Geometry check sheet. Reference: the model listing, model coordinates, mm. A direction names the side the tool comes from. Round coordinates to 2 decimals unless told otherwise and drop trailing zeros. Write each loop counter-clockwise with the first axis right and the second up, starting at its lowest first coordinate (ties: lowest second). Pieces come first, ordered by that corner, then holes. Notation, with made-up numbers: M 8.25,10.25 L 66.25,10.25 A25 ccw 66.25,29.25 Z; hole C 61.5,10 d11. An arc over 180 degrees is marked long. Use a Markdown table: item, result.
```python
from build123d import *

# Parameters (mm, degrees)
BOSS_EXTRUDE1_DEPTH  = 1.5875
M4_CLEARANCE_HOLE1_D = 4.5
BOSS_EXTRUDE2_DEPTH  = 3.175
M3_CLEARANCE_HOLE1_D = 3.4
FILLET1_R            = 3.5
SKETCH8_R            = 2.15
CUT_EXTRUDE1_DEPTH   = 4.1750001
SKETCH9_R            = 2.75
SKETCH9_R_2          = 2.15
BOSS_EXTRUDE3_DEPTH  = 0.75
SKETCH11_R           = 3.5
CUT_EXTRUDE2_DEPTH   = 2.5
SKETCH12_R           = 2.75
CUT_EXTRUDE3_DEPTH   = 0.2
SKETCH13_R           = 3
SKETCH13_R_2         = 2.25
BOSS_EXTRUDE5_DEPTH  = 1.5


with BuildPart() as part:
    # Sketch2 → Boss-Extrude1 (new body, symmetric)
    with BuildSketch(Plane.XY):
        with BuildLine():
            add(Edge.make_bspline(
                [(-24.777431429, -6.350183234), (-24.299810251, -5.902972393), (-23.32289496, -5.01651393), (-22.058866471, -3.944003435), (-21.276036232, -3.316259916), (-20.98344634, -3.086723573)],
                knots=[0, 0, 0, 0, 0.03125, 0.0625, 0.081068463, 0.081068463, 0.081068463, 0.081068463], degree=3))
            Line((-24.777431429, -6.350183234), (-21.36, -10))
            add(Edge.make_bspline(
                [(-21.36, -10), (-20.09052587, -8.81135381), (-18.821051739, -7.728673603), (-17.551577609, -6.751959378)],
                knots=[0, 0, 0, 0, 0.089148464, 0.089148464, 0.089148464, 0.089148464], degree=3))
            Line((-17.551577609, -6.751959378), (-20.98344634, -3.086723573))
        make_face()
        with BuildLine():
            Line((-21.36, -10), (-24.777431429, -6.350183234))
            ThreePointArc((-24.777431429, -6.350183234), (-26.357299125, -9.8356788), (-25.009816701, -13.417431499))
            ThreePointArc((-25.009816701, -13.417431499), (-21.5243212, -14.997299125), (-17.942568571, -13.649816766))
            Line((-17.942568571, -13.649816766), (-21.36, -10))
        make_face()
        with BuildLine():
            ThreePointArc((-25.009816701, -13.417431499), (-26.357299125, -9.8356788), (-24.777431429, -6.350183234))
            add(Edge.make_bspline(
                [(-24.777431429, -6.350183234), (-24.299810251, -5.902972393), (-23.32289496, -5.01651393), (-22.058866471, -3.944003435), (-21.276036232, -3.316259916), (-20.98344634, -3.086723573)],
                knots=[0, 0, 0, 0, 0.03125, 0.0625, 0.081068463, 0.081068463, 0.081068463, 0.081068463], degree=3))
            Line((-20.98344634, -3.086723573), (-21.127614663, -2.932751805))
            Line((-21.127614663, -2.932751805), (-23.519816663, -0.377880068))
            ThreePointArc((-23.519816663, -0.377880068), (-30.587064859, -0.145494731), (-30.819450196, -7.212742926))
            Line((-30.819450196, -7.212742926), (-28.427248195, -9.767614663))
            Line((-28.427248195, -9.767614663), (-25.009816701, -13.417431499))
        make_face()
        with BuildLine():
            add(Edge.make_bspline(
                [(-21.36, -10), (-20.09052587, -8.81135381), (-18.821051739, -7.728673603), (-17.551577609, -6.751959378)],
                knots=[0, 0, 0, 0, 0.089148464, 0.089148464, 0.089148464, 0.089148464], degree=3))
            Line((-21.36, -10), (-17.942568571, -13.649816766))
            add(Edge.make_bspline(
                [(-17.942568571, -13.649816766), (-17.543072686, -13.275756949), (-16.7212792, -12.530114496), (-15.44829951, -11.450473224), (-14.582019434, -10.770813046), (-14.116024052, -10.421130577)],
                knots=[0, 0, 0, 0, 0.03125, 0.0625, 0.099339971, 0.099339971, 0.099339971, 0.099339971], degree=3))
            Line((-14.116024052, -10.421130577), (-14.292751805, -10.232385337))
            Line((-14.292751805, -10.232385337), (-17.551577609, -6.751959378))
        make_face()
        with BuildLine():
            ThreePointArc((-17.942568571, -13.649816766), (-21.5243212, -14.997299125), (-25.009816701, -13.417431499))
            Line((-25.009816701, -13.417431499), (-21.592385337, -17.067248195))
            Line((-21.592385337, -17.067248195), (-19.200183337, -19.622119932))
            ThreePointArc((-19.200183337, -19.622119932), (-12.132935141, -19.854505269), (-11.900549804, -12.787257074))
            Line((-11.900549804, -12.787257074), (-14.116024052, -10.421130577))
            add(Edge.make_bspline(
                [(-17.942568571, -13.649816766), (-17.543072686, -13.275756949), (-16.7212792, -12.530114496), (-15.44829951, -11.450473224), (-14.582019434, -10.770813046), (-14.116024052, -10.421130577)],
                knots=[0, 0, 0, 0, 0.03125, 0.0625, 0.099339971, 0.099339971, 0.099339971, 0.099339971], degree=3))
        make_face()
        with BuildLine():
            add(Edge.make_bspline(
                [(-20.98344634, -3.086723573), (-20.291201445, -2.543658465), (-18.603117827, -1.28817338), (-15.885096675, 0.462779531), (-11.785009924, 2.624744664), (-6.509375137, 4.48808894), (0, 5.25595553), (6.509375137, 4.48808894), (11.785009924, 2.624744664), (15.885096675, 0.462779531), (18.901874802, -1.480633029), (21.37388106, -3.362802893), (23.32289496, -5.01651393), (24.299810251, -5.902972393), (24.777431429, -6.350183234)],
                knots=[0.081068463, 0.081068463, 0.081068463, 0.081068463, 0.125, 0.1875, 0.25, 0.375, 0.5, 0.625, 0.75, 0.8125, 0.875, 0.9375, 0.96875, 1, 1, 1, 1], degree=3))
            Line((-20.98344634, -3.086723573), (-17.551577609, -6.751959378))
            Line((-17.551577609, -6.751959378), (-14.292751805, -10.232385337))
            Line((-14.292751805, -10.232385337), (-14.116024052, -10.421130577))
            add(Edge.make_bspline(
                [(-14.116024052, -10.421130577), (-13.791445759, -10.177567349), (-12.680801028, -9.370838959), (-10.815202086, -8.171392792), (-7.794818062, -6.582915934), (-4.170679183, -5.321481205), (0, -4.839259398), (4.170679183, -5.321481205), (7.794818062, -6.582915934), (10.815202086, -8.171392792), (13.136984474, -9.664132159), (15.119482265, -11.171596294), (16.7212792, -12.530114496), (17.543072686, -13.275756949), (17.942568571, -13.649816766)],
                knots=[0.099339971, 0.099339971, 0.099339971, 0.099339971, 0.125, 0.1875, 0.25, 0.375, 0.5, 0.625, 0.75, 0.8125, 0.875, 0.9375, 0.96875, 1, 1, 1, 1], degree=3))
            ThreePointArc((17.942568571, -13.649816766), (25.009816766, -13.417431429), (24.777431429, -6.350183234))
        make_face()
    extrude(amount=BOSS_EXTRUDE1_DEPTH, both=True)

    # M4 Clearance Hole1 (through all)
    with Locations(Plane.XY.offset(1.5875)):
        with Locations((-21.359999999, -9.999999999), (0, 0), (-15.550366571, -16.204688503), (-27.169633429, -3.795311497)):
            Hole(M4_CLEARANCE_HOLE1_D / 2)

    # Sketch5 → Boss-Extrude2 (add)
    with BuildSketch(Plane(origin=(0, 0, -1.5875), x_dir=(-1, 0, 0), z_dir=(0, 0, -1))):
        with BuildLine():
            ThreePointArc((-23.201229183, -22.868950039), (-17.11, -26.460179221), (-13.518770817, -20.368950039))
            Line((-13.518770817, -20.368950039), (-16.518770817, -8.75))
            ThreePointArc((-16.518770817, -8.75), (-22.61, -5.158770817), (-26.201229183, -11.25))
            Line((-26.201229183, -11.25), (-23.201229183, -22.868950039))
        make_face()
    extrude(amount=-BOSS_EXTRUDE2_DEPTH)

    # M3 Clearance Hole1 (through all)
    with Locations(Plane(origin=(0, 0, -1.5875), x_dir=(-1, 0, 0), z_dir=(0, 0, -1))):
        with Locations((-18.36, -21.618950039)):
            Hole(M3_CLEARANCE_HOLE1_D / 2)

    # Fillet1
    fillet1_edges = [part.edges().sort_by_distance(p)[0] for p in [
        (15.75315909, -11.715201468, -0.79375),
        (-20.98344634, -3.086723573, -0.79375),
        (-14.116024052, -10.421130577, 0.79375),
    ]]
    fillet(fillet1_edges, radius=FILLET1_R)

    # Sketch8 → Cut-Extrude1 (cut, through all)
    with BuildSketch(Plane(origin=(0, 0, -1.5875), x_dir=(-1, 0, 0), z_dir=(0, 0, -1))):
        with Locations((-21.36, -10)):
            Circle(SKETCH8_R)
    extrude(amount=-CUT_EXTRUDE1_DEPTH, mode=Mode.SUBTRACT)

    # Sketch9 → Boss-Extrude3 (add)
    with BuildSketch(Plane(origin=(0, 0, -1.5875), x_dir=(-1, 0, 0), z_dir=(0, 0, -1))):
        with Locations((-21.36, -10)):
            Circle(SKETCH9_R)
        with Locations((-21.36, -10)):
            Circle(SKETCH9_R_2, mode=Mode.SUBTRACT)
    extrude(amount=BOSS_EXTRUDE3_DEPTH)

    # Sketch11 → Cut-Extrude2 (cut)
    with BuildSketch(Plane.XY.offset(1.5875)):
        with Locations((-21.359999999, -9.999999999)):
            Circle(SKETCH11_R)
    extrude(amount=-CUT_EXTRUDE2_DEPTH, mode=Mode.SUBTRACT)

    # Sketch12 → Cut-Extrude3 (cut)
    with BuildSketch(Plane.XY.offset(-0.9125)):
        with Locations((-21.359999999, -9.999999999)):
            Circle(SKETCH12_R)
    extrude(amount=-CUT_EXTRUDE3_DEPTH, mode=Mode.SUBTRACT)

    # Sketch13 → Boss-Extrude5 (add)
    with BuildSketch(Plane(origin=(0, 0, -1.5875), x_dir=(-1, 0, 0), z_dir=(0, 0, -1))):
        with Locations((21.359999999, -9.999999999)):
            Circle(SKETCH13_R)
        with Locations((21.359999999, -9.999999999)):
            Circle(SKETCH13_R_2, mode=Mode.SUBTRACT)
    extrude(amount=BOSS_EXTRUDE5_DEPTH)


solid = part.part
```
Item 1: Mould release check, pull along Y, two halves, no side actions. Record for faces 4 (the face through (-23.5, -9.3, -2.1)), 5 (the face through (20, -12, -2.338)), 6 (the face through (24.72, -16.98, -0.02)), 7 (the face through (-30.506, -0.071, 0.022)): +Y half, -Y half, draft (parallel to the pull), parting line (faces both ways), or undercut.
Outcome:
| item | result |
|---|---|
| face 4 | undercut |
| face 5 | draft |
| face 6 | -Y half |
| face 7 | parting line |
Item 2: Go/stop test with flat-tipped pins: pin 1 (2 mm diameter, centred on x = 7.5, z = -0.5, fed in from -Y); pin 2 (5 mm diameter, centred on x = -15.55, y = -16.2, fed in from -Z); pin 3 (1.5 mm diameter, centred on y = -18.5, z = -2, fed in from +X). Record where each tip stops, or that it passes through.
Outcome:
| item | result |
|---|---|
| pin 1 | stops at y = -7 |
| pin 2 | stops at z = -1.59 |
| pin 3 | stops at x = 24.49 |
Item 3: Cross-section at B-B, the plane z = 0.75. Count the separate pieces of the cut face and the enclosed holes in it, and give its area (3 significant figures).
Outcome:
| item | result |
|---|---|
| separate pieces | 1 |
| enclosed holes | 6 |
| area | 736 mm2 |
Item 4: Access from +Z, -Z, +X, -X, +Y, -Y to the whole of each face (thin tool, end or side, straight path). Record for faces 1 (the face through (-24.13, -11.15, -2.33)), 2 (the face through (-24.857, -9.846, 0.355)), 3 (the face through (14.34, -17.19, -0.02)).
Outcome:
| item | result |
|---|---|
| face 1 | -Z |
| face 2 | +Z |
| face 3 | +Z, -Z |
Item 5: Material ranges on line 1 along Y through (x, z) = (-21.36, -2.3); line 2 along X through (y, z) = (-14.5, -0.4); line 3 along Y through (x, z) = (-28, -0.25), recorded low to high. Write a range as from..to.
Outcome:
| item | result |
|---|---|
| line 1 | y = -13..-12.25, -7.75..-7 |
| line 2 | x = -24..-17.02, -14.08..-10.85, 15.03..25.36 |
| line 3 | y = -10.22..-5.89, -1.7..1.14 |
Item 6: Cross-section at A-A, the plane y = -19. Record the cut outline in (x, z).
Outcome:
| item | result |
|---|---|
| outline | M -19.78,-1.59 L -11.4,-1.59 L -11.4,1.59 L -19.78,1.59 Z; M 13.87,-1.59 L 24.2,-1.59 L 24.2,1.59 L 13.87,1.59 Z |
